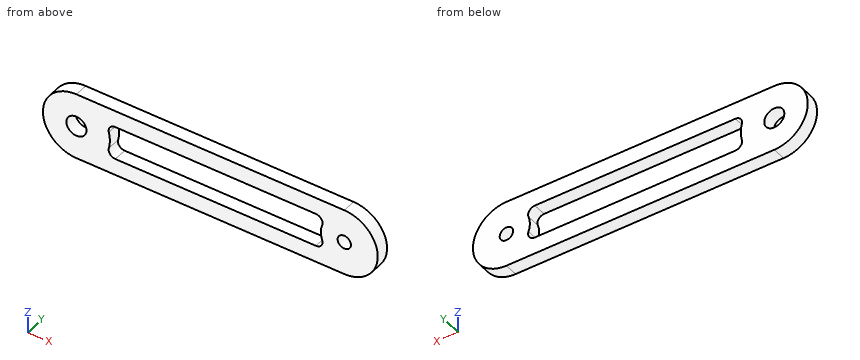
```python
from build123d import *

# Parameters (mm, degrees)
BOSS_EXTRUDE1_DEPTH = 2
SKETCH4_R           = 1
CUT_EXTRUDE3_DEPTH  = 12.7
SKETCH5_R           = 1.5
CUT_EXTRUDE4_DEPTH  = 10
CUT_EXTRUDE5_REACH  = 27.573


with BuildPart() as part:
    # Sketch1 → Boss-Extrude1 (new body)
    with BuildSketch(Plane(origin=(0, 0, 0), x_dir=(1, 0, 0), z_dir=(0, 1, 0))):
        with BuildLine():
            Line((-20, 5), (20, 5))
            ThreePointArc((20, 5), (25, 0), (20, -5))
            Line((20, -5), (-20, -5))
            ThreePointArc((-20, -5), (-25, 0), (-20, 5))
        make_face()
    extrude(amount=BOSS_EXTRUDE1_DEPTH)

    # Sketch4 → Cut-Extrude3 (cut)
    with BuildSketch(Plane(origin=(0, 2, 0), x_dir=(1, 0, 0), z_dir=(0, 1, 0))):
        with Locations(Location((20, 0, 0), (0, 0, 270))):
            Circle(SKETCH4_R)
    extrude(amount=-CUT_EXTRUDE3_DEPTH, mode=Mode.SUBTRACT)

    # Sketch5 → Cut-Extrude4 (cut)
    with BuildSketch(Plane(origin=(0, 2, 0), x_dir=(1, 0, 0), z_dir=(0, 1, 0))):
        with Locations(Location((-20, 0, 0), (0, 0, 270))):
            Circle(SKETCH5_R)
    extrude(amount=-CUT_EXTRUDE4_DEPTH, mode=Mode.SUBTRACT)

    # Sketch6 → Cut-Extrude5 (cut, up to next)
    with BuildSketch(Plane.XZ, mode=Mode.PRIVATE) as cut_extrude5_sk1:
        with BuildLine():
            Line((15.757359313, -2.5), (-14.190524981, -2.5))
            ThreePointArc((-14.190524981, -2.5), (-14.981094396, -2.112372436), (-15.158770817, -1.25))
            ThreePointArc((-15.158770817, -1.25), (-15, 0), (-15.158770817, 1.25))
            ThreePointArc((-15.158770817, 1.25), (-14.981094396, 2.112372436), (-14.190524981, 2.5))
            Line((-14.190524981, 2.5), (15.757359313, 2.5))
            ThreePointArc((15.757359313, 2.5), (16.573855894, 2.077350269), (16.700168354, 1.166666667))
            ThreePointArc((16.700168354, 1.166666667), (16.5, 0), (16.700168354, -1.166666667))
            ThreePointArc((16.700168354, -1.166666667), (16.573855894, -2.077350269), (15.757359313, -2.5))
        make_face()
    cut_extrude5_tool1 = extrude(cut_extrude5_sk1.sketch, amount=-CUT_EXTRUDE5_REACH, mode=Mode.PRIVATE) & part.part
    add(cut_extrude5_tool1.solids().sort_by_distance((0.772522, 0, 0))[0], mode=Mode.SUBTRACT)


solid = part.part
```
The listing builds one solid part. Answer for the finished solid, in the listing's coordinates (mm). Give positions to 0.01 mm unless a question says otherwise; leave off trailing zeros. Write each loop counter-clockwise with the first axis right and the second up, starting at its lowest first coordinate (ties: lowest second). Pieces come first, ordered by that corner, then holes. Notation, with made-up numbers: (-16, 44) - (22, 44) arc R19 ccw to (22, 50) - close; hole circle Ø6 at (14.25, 5). An arc over 180 degrees is marked (long way). Use one line per item in the form item = value. Start each with the question number.
1) Find section B-B on y = 0.85. Determine the outline of the cut face in (x, z), plus the area to 3 significant figures.
2) Find section A-A on x = 4.5. Determine the outline of the cut face in (y, z).
3) Find section C-C on z = 0. Determine the outline of the cut face in (x, y), plus the area to 3 significant figures.
4) Consider line 1 along X through (y, z) = (0.55, 0); line 2 along Z through (x, y) = (11, 0.65); line 3 along X through (y, z) = (0.95, 2). Determine where each line is inside the solid, lowest interval first. Write a range as from..to.
5) Find section D-D on z = 2. Determine the outline of the cut face in (x, y), plus the area to 3 significant figures.
Geometry results:
q1.outline = (-20, -5) - (20, -5) arc R5 ccw to (20, 5) - (-20, 5) arc R5 ccw to start; hole circle Ø3 at (-20, 0); hole (-15.16, -1.25) arc R1 ccw to (-14.19, -2.5) - (15.76, -2.5) arc R1 ccw to (16.7, -1.17) arc R3.5 cw to (16.7, 1.17) arc R1 ccw to (15.76, 2.5) - (-14.19, 2.5) arc R1 ccw to (-15.16, 1.25) arc R5 cw to start; hole circle Ø2 at (20, 0)
q1.area = 310 mm2
q2.outline = (0, -5) - (2, -5) - (2, -2.5) - (0, -2.5) - close; (0, 2.5) - (2, 2.5) - (2, 5) - (0, 5) - close
q3.outline = (-25, 0) - (-21.5, 0) - (-21.5, 2) - (-25, 2) - close; (-18.5, 0) - (-15, 0) - (-15, 2) - (-18.5, 2) - close; (16.5, 0) - (19, 0) - (19, 2) - (16.5, 2) - close; (21, 0) - (25, 0) - (25, 2) - (21, 2) - close
q3.area = 27.0 mm2
q4.line_1 = -25..-21.5, -18.5..-15, 16.5..19, 21..25
q4.line_2 = -5..-2.5, 2.5..5
q4.line_3 = -24.58..-15.06, 16.62..24.58
q5.outline = (-24.58, 0) - (-15.06, 0) - (-15.06, 2) - (-24.58, 2) - close; (16.62, 0) - (24.58, 0) - (24.58, 2) - (16.62, 2) - close
q5.area = 35.0 mm2
